Design review of the part built by this model. Coordinates are the model's own, in mm. A direction names the side the tool comes from. Coordinates: 2 decimals unless noted, no trailing zeros. Write each loop counter-clockwise with the first axis right and the second up, starting at its lowest first coordinate (ties: lowest second). Pieces come first, ordered by that corner, then holes. Notation, with made-up numbers: M -20,70.5 L 8,70.5 A28 ccw 8,94.5 Z; hole C 3.5,59 d2. An arc over 180 degrees is marked long. Write item = value, one per line.
```python
from build123d import *

# Parameters (mm, degrees)
F1_DEPTH = 5
F2_W     = 1
F2_H     = 1
F3_DEPTH = 1
F4_W     = 1
F4_H     = 1
F5_DEPTH = 1


with BuildPart() as f1:
    # F0 (on Top) → F1 (new body)
    with BuildSketch(Plane.XY):
        Polygon((13.737387, -5), (0, 0), (13.737387, 5), (58.737387, 5), (58.737387, 6), (13.737387, 6), (0, 1), (-5, 1), (-5, -1), (0, -1), (13.737387, -6), (63.737387, -6), (63.737387, -5), align=None)
    extrude(amount=F1_DEPTH)

    # F2 (on face) → F3 (cut, through all)
    with BuildSketch(Plane(origin=(0, 6, 0), x_dir=(-1, 0, 0), z_dir=(0, 1, 0))):
        with Locations((-57.237387, 4.5)):
            Rectangle(F2_W, F2_H)
        with Locations((-57.237387, 0.5)):
            Rectangle(F2_W, F2_H)
    extrude(amount=-F3_DEPTH, mode=Mode.SUBTRACT)

    # F4 (on face) → F5 (cut, through all)
    with BuildSketch(Plane.XZ.offset(6)):
        with Locations((62.237387, 4.5)):
            Rectangle(F4_W, F4_H)
        with Locations((62.237387, 0.5)):
            Rectangle(F4_W, F4_H)
    extrude(amount=-F5_DEPTH, mode=Mode.SUBTRACT)


solid = f1.part
```
Q1. Consider section B-B, the plane z = 2.1. State the section outline as (x, y) points, and give its area (3 significant figures).
Check result:
outline = M -5,-1 L 0,-1 L 13.74,-6 L 63.74,-6 L 63.74,-5 L 13.74,-5 L 0,0 L 13.74,5 L 58.74,5 L 58.74,6 L 13.74,6 L 0,1 L -5,1 Z
area = 132 mm²
Q2. Consider section C-C, the plane y = 3.25. State the section outline as (x, z) points.
Check result:
outline = M 6.18,0 L 8.93,0 L 8.93,5 L 6.18,5 Z
Q3. Consider section A-A, the plane x = 38.5. State the section outline as (y, z) points, and give its area (3 significant figures).
Check result:
outline = M -6,0 L -5,0 L -5,5 L -6,5 Z; M 5,0 L 6,0 L 6,5 L 5,5 Z
area = 10.0 mm²
Q4. Wall thickness on line 1 (Y direction, x = 39.5, z = 1.2); line 2 (Y direction, x = 11, z = 3.9): over which ranges is each line inside the solid? List them lowest first.
Check result:
line_1 = -6 to -5, 5 to 6
line_2 = -5 to -4, 4 to 5
Q5. Machinability: for faces 1 (the flat face through (-3, -1, 2)), 2 (the flat face through (-5, 0, 2)), 3 (the flat face through (-2, 1, 2)), 4 (the flat face through (39, -5, 2)), which of the approach directions +Z, -Z, +X, -X, +Y, -Y give a long, thin tool a straight path to every point of the face, cutting with its end or side? Answer none if there is none.
Check result:
face_1 = +Z, -Z, -X, -Y
face_2 = +Z, -Z, -X, +Y, -Y
face_3 = +Z, -Z, -X, +Y
face_4 = +Z, -Z, +X
Q6. For P1, Ø1.5, axis at x = -3.5, z = 2.5, coming from the -Y side; P2, Ø0.5, axis at y = 5.5, z = 0.5, coming from the +X side; P3, Ø1.5, axis at x = -3.5, z = 2, coming from the +Y side, all flat-tipped, find the tip position at first contact; note any pin that passes through.
Check result:
P1 = -1
P2 = 58.74
P3 = 1
